```python
from build123d import *


with BuildPart() as part:
    # Sketch1 → Revolve1 (revolve)
    with BuildSketch(Plane(origin=(0, 0, 0), x_dir=(0, 0, -1), z_dir=(1, 0, 0)), mode=Mode.PRIVATE) as revolve1_sk:
        with BuildLine():
            Line((0, 2.45), (0, 4.25))
            Line((0, 4.25), (-5, 4.25))
            Line((-5, 4.25), (-5, 7.738899697))
            ThreePointArc((-5, 7.738899697), (-4.867562217, 8.077865797), (-4.540407934, 8.237264222))
            Line((-4.540407934, 8.237264222), (6.1, 9.1))
            Line((6.1, 9.1), (6.1, 2.85))
            Line((6.1, 2.85), (3.8, 2.85))
            Line((3.8, 2.85), (3.8, 2.45))
            Line((3.8, 2.45), (0, 2.45))
        make_face()
    revolve(revolve1_sk.sketch.rotate(Axis((0, 0, 0), (0, 0, 1)), 90), axis=Axis((0, 0, 0), (0, 0, 1)))


solid = part.part
```
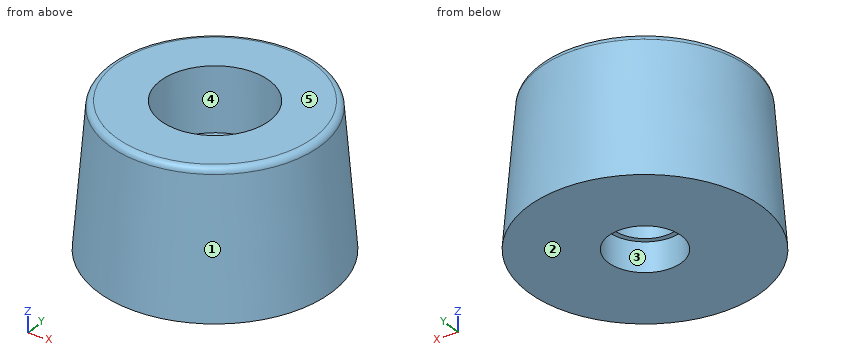
Work out the finished part from the listing and answer in its coordinate system (mm). Face numbers are marked on the shaded views. A direction names the side the tool comes from. Give positions to 0.01 mm unless a question says otherwise; leave off trailing zeros. Loops run counter-clockwise (first coordinate to the right, second up) from the corner with the lowest first, then second, coordinate; pieces in that order, holes last. Notation, with made-up numbers: (-39.75, -1) - (-12.75, -1) arc R31 cw to (-12.75, 30) - close; hole circle Ø6 at (29.5, -1). An arc over 180 degrees is marked (long way). One line per question, with ' | ' between items.
(1) The mould has two halves that part along Y. Classify the marked faces 1, 2 and 3: +Y half, -Y half, draft (parallel to the pull), parting line (faces both ways), or undercut.
Recorded:
face 1: parting line | face 2: draft | face 3: undercut
(2) The part is cut by section C-C (z = -3). Write down the section's boundary in (x, y), then the cut area to 3 significant figures.
Recorded:
outline: circle Ø17.7 at (0, 0); hole circle Ø4.9 at (0, 0) | area: 227 mm²
(3) The part is cut by section D-D (z = 2.25). Write down the section's boundary in (x, y), then the cut area to 3 significant figures.
Recorded:
outline: circle Ø16.85 at (0, 0); hole circle Ø8.5 at (0, 0) | area: 166 mm²
(4) A tool of negligible diameter and unlimited length cuts with its end or side. For the marked faces 4 and 5, from which of +Z, -Z, +X, -X, +Y, -Y can it reach the whole face along a straight path? Write none if from no direction.
Recorded:
face 4: +Z | face 5: +Z, +X, -X, +Y, -Y
(5) The part is cut by section A-A (x = 0). Write down the section's boundary in (y, z).
Recorded:
outline: (-9.1, -6.1) - (-2.85, -6.1) - (-2.85, -3.8) - (-2.45, -3.8) - (-2.45, 0) - (-4.25, 0) - (-4.25, 5) - (-7.74, 5) arc R0.5 ccw to (-8.24, 4.54) - close; (2.45, -3.8) - (2.85, -3.8) - (2.85, -6.1) - (9.1, -6.1) - (8.24, 4.54) arc R0.5 ccw to (7.74, 5) - (4.25, 5) - (4.25, 0) - (2.45, 0) - close
(6) Each of these flat-tipped pins is pushed along its axis until it touches: pin 1 Ø7 at (x, y) = (0, 0) entering from +Z; pin 2 Ø2 at (x, y) = (-0.5, -0.5) entering from -Z; pin 3 Ø4 at (y, z) = (6, 0) entering from +X; pin 4 Ø3 at (x, z) = (-6.5, 1.5) entering from +Y. Where does it stop, or does it pass through?
Recorded:
pin 1: stops at z = 0 | pin 2: passes through | pin 3: stops at x = 7.64 | pin 4: stops at y = 6.86
(7) Straight lines are drawn through the part: probe 1 along Y at (x, z) = (0, -2.85); probe 2 along Y at (x, z) = (0, -4.6); probe 3 along Z at (x, y) = (3.5, 1). For each, find the intervals that lie inside material, in ascending order.
Recorded:
probe 1: y = -8.84 to -2.45, 2.45 to 8.84 | probe 2: y = -8.98 to -2.85, 2.85 to 8.98 | probe 3: z = -6.1 to 0
